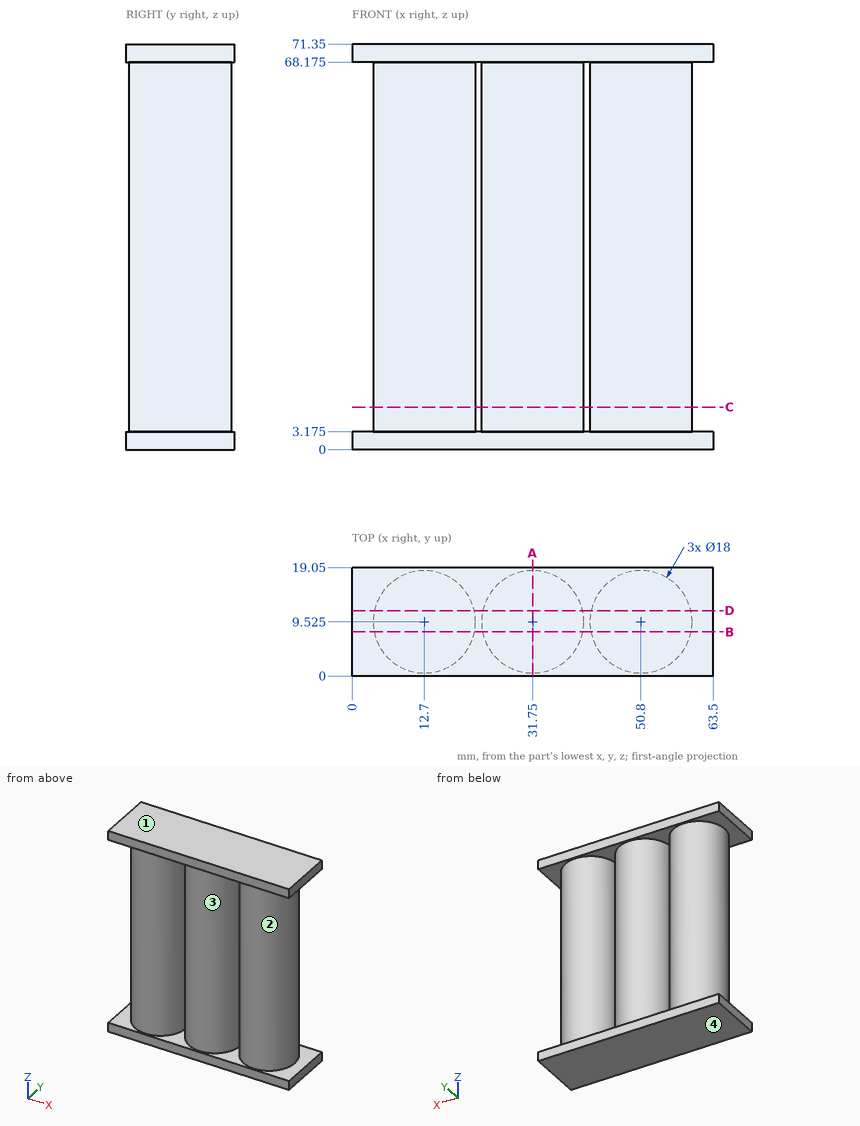
Could you check a few things on this drawing? It's one solid part, dimensions in mm from its lowest x, y, z. A direction names the side the tool comes from. Round coordinates to 2 decimals unless told otherwise and drop trailing zeros. Loops run counter-clockwise (first coordinate to the right, second up) from the corner with the lowest first, then second, coordinate; pieces in that order, holes last. Notation, with made-up numbers: M 19,-21.5 L 32,-21.5 A31 cw 32,13.5 Z; hole C -8.5,-10.75 d11. An arc over 180 degrees is marked long. Write each question's results on one line, items separated by ' | '. Start each with the question number.
(1) Will these pins go through, and if not, where does the flat tip stop? P1, Ø5, axis at y = 6.5, z = 63.5, coming from the -X side; P2, Ø1, axis at x = 23, z = 58, coming from the -Y side; P3, Ø8, axis at y = 2.5, z = 57, coming from the -X side.
(2) If I drill on probe 1 along X at (y, z) = (9.75, 5); probe 2 along X at (y, z) = (16, 16); probe 3 along Y at (x, z) = (49, 66.5), over which ranges is the centre line in solid material (lowest first)? Write a range as from..to.
(3) On a 3-axis mill with a long thin cutter (end or side, diameter ignored), from which of +Z, -Z, +X, -X, +Y, -Y can I reach the whole of each face in a straight line? I mean the marked faces 3 and 4. Say none if no direction works.
(4) I want a section at B-B (y = 7.75). Please give me the cut outline in (x, z) (3 decimals), then the cut area to 3 significant figures.
(5) Thinking about a two-plate mould opening in X: for the marked faces 1 and 2, which applies, pulls with the +X half, pulls with the -X half, needs draft (parallel to the pull), parting line crosses it, or undercut?
(6) I want a section at A-A (x = 31.75). Please give me the cut outline in (y, z) (3 decimals), then the cut area to 3 significant figures.
(7) I want a section at D-D (y = 11.5). Please give me the cut outline in (x, z) (3 decimals).
(8) I want a section at C-C (z = 7.5). Please give me the cut outline in (x, y) (3 decimals).
Solved:
1) P1: stops at x = 3.72 | P2: stops at y = 5.93 | P3: stops at x = 4.22
2) probe 1: x = 3.7..21.7, 22.75..40.75, 41.8..59.8 | probe 2: x = 6.45..18.95, 25.5..38, 44.55..57.05 | probe 3: y = 0.71..18.34
3) face 3: none | face 4: -Z, +X, -X, +Y, -Y
4) outline: M 0,0 L 63.5,0 L 63.5,3.175 L 59.623,3.175 L 59.623,68.175 L 63.5,68.175 L 63.5,71.35 L 0,71.35 L 0,68.175 L 3.877,68.175 L 3.877,3.175 L 0,3.175 Z; hole M 21.523,3.175 L 22.927,3.175 L 22.927,68.175 L 21.523,68.175 Z; hole M 40.573,3.175 L 41.977,3.175 L 41.977,68.175 L 40.573,68.175 Z | area: 3,840 mm²
5) face 1: needs draft | face 2: undercut
6) outline: M 0,0 L 19.05,0 L 19.05,3.175 L 18.525,3.175 L 18.525,68.175 L 19.05,68.175 L 19.05,71.35 L 0,71.35 L 0,68.175 L 0.525,68.175 L 0.525,3.175 L 0,3.175 Z | area: 1,290 mm²
7) outline: M 0,0 L 63.5,0 L 63.5,3.175 L 59.581,3.175 L 59.581,68.175 L 63.5,68.175 L 63.5,71.35 L 0,71.35 L 0,68.175 L 3.919,68.175 L 3.919,3.175 L 0,3.175 Z; hole M 21.481,3.175 L 22.969,3.175 L 22.969,68.175 L 21.481,68.175 Z; hole M 40.531,3.175 L 42.019,3.175 L 42.019,68.175 L 40.531,68.175 Z
8) outline: C 12.7,9.525 d18; C 31.75,9.525 d18; C 50.8,9.525 d18
